from build123d import *

# Parameters (mm, degrees)
SKETCH1_W           = 19.7
SKETCH1_H           = 5.7
SKETCH1_R           = 1.125
BOSS_EXTRUDE1_DEPTH = 0.6
SKETCH2_W           = 10.7
SKETCH2_H           = 5.7
BOSS_EXTRUDE2_DEPTH = 5
SKETCH3_W           = 3.05
SKETCH3_H           = 3.05
BOSS_EXTRUDE3_DEPTH = 7
BOSS_EXTRUDE4_DEPTH = 5


with BuildPart() as part:
    # Sketch1 → Boss-Extrude1 (new body)
    with BuildSketch(Plane.XY):
        with Locations((0, -89.5)):
            Rectangle(SKETCH1_W, SKETCH1_H)
        with Locations((7.5, -89.5)):
            Circle(SKETCH1_R, mode=Mode.SUBTRACT)
        with Locations((-7.5, -89.5)):
            Circle(SKETCH1_R, mode=Mode.SUBTRACT)
    extrude(amount=BOSS_EXTRUDE1_DEPTH)

    # Sketch2 → Boss-Extrude2 (add)
    with BuildSketch(Plane.XY.offset(0.6)):
        with Locations((0, -89.5)):
            Rectangle(SKETCH2_W, SKETCH2_H)
    extrude(amount=BOSS_EXTRUDE2_DEPTH)

    # Sketch3 → Boss-Extrude3 (add)
    with BuildSketch(Plane(origin=(0, 0, 0), x_dir=(-1, 0, 0), z_dir=(0, 0, -1))):
        with Locations((-1.525, -89.5)):
            Rectangle(SKETCH3_W, SKETCH3_H)
    extrude(amount=BOSS_EXTRUDE3_DEPTH)

    # Sketch4 → Boss-Extrude4 (add)
    with BuildSketch(Plane.XY.offset(5.6)):
        with BuildLine():
            Line((-0.5, -89.25), (0.5, -89.25))
            ThreePointArc((0.5, -89.25), (0.75, -89.5), (0.5, -89.75))
            Line((0.5, -89.75), (-0.5, -89.75))
            ThreePointArc((-0.5, -89.75), (-0.75, -89.5), (-0.5, -89.25))
        make_face()
        with BuildLine():
            Line((2, -89.25), (3, -89.25))
            ThreePointArc((3, -89.25), (3.25, -89.5), (3, -89.75))
            Line((3, -89.75), (2, -89.75))
            ThreePointArc((2, -89.75), (1.75, -89.5), (2, -89.25))
        make_face()
        with BuildLine():
            Line((-3, -89.25), (-2, -89.25))
            ThreePointArc((-2, -89.25), (-1.75, -89.5), (-2, -89.75))
            Line((-2, -89.75), (-3, -89.75))
            ThreePointArc((-3, -89.75), (-3.25, -89.5), (-3, -89.25))
        make_face()
    extrude(amount=BOSS_EXTRUDE4_DEPTH)


solid = part.part
Geometry: final body of the model. Coordinates: model frame, mm. A direction names the side the tool comes from. Round coordinates to 2 decimals unless told otherwise and drop trailing zeros. Write each loop counter-clockwise with the first axis right and the second up, starting at its lowest first coordinate (ties: lowest second). Pieces come first, ordered by that corner, then holes. Notation, with made-up numbers: M 33,77 L 87,77 A18 cw 87,108 Z; hole C -14,-39.5 d11. An arc over 180 degrees is marked long. Write item = value, one per line.
Item 1: Section query A-A on x = -7.5. Return loops of the section in (y, z) (3 decimals), then the cut area to 3 significant figures.
Findings:
outline = M -92.35,0 L -90.625,0 L -90.625,0.6 L -92.35,0.6 Z; M -88.375,0 L -86.65,0 L -86.65,0.6 L -88.375,0.6 Z
area = 2.07 mm^2
Item 2: Pin query (flat end, axial travel): P1, Ø4, axis at x = -2.5, z = -4, coming from the +Y side; P2, Ø0.5, axis at x = 2.5, z = 7, coming from the +Y side; P3, Ø2.5, axis at y = -88.5, z = 3.5, coming from the -X side; P4, Ø1.5, axis at x = -7.5, y = -88, coming from the +Z side. Return the tip coordinate at first contact, or that it passes through.
Findings:
P1 = through
P2 = -89.25
P3 = -5.35
P4 = 0.6
Item 3: Access query for faces 1 (the face through (0, -89.25, 8)), 2 (the face through (5.35, -90, 3)), 3 (the face through (-9, -89, 0.6)). Directions: +Z, -Z, +X, -X, +Y, -Y. A direction counts if a zero-diameter tool reaches every point of the face in a straight line with its end or side. Return the directions, or none.
Findings:
face_1 = +Z, +X, -X, +Y
face_2 = +Z, +X, +Y, -Y
face_3 = +Z, -X, +Y, -Y
Item 4: Section query C-C on z = 2.5. Return loops of the section in (x, y), then the cut area to 3 significant figures.
Findings:
outline = M -5.35,-92.35 L 5.35,-92.35 L 5.35,-86.65 L -5.35,-86.65 Z
area = 61.0 mm^2
Item 5: Section query D-D on x = 4. Return loops of the section in (y, z), then the cut area to 3 significant figures.
Findings:
outline = M -92.35,0 L -86.65,0 L -86.65,5.6 L -92.35,5.6 Z
area = 31.9 mm^2
Item 6: Material intervals for line 1 along X through (y, z) = (-89.5, 0.2) (3 decimals); line 2 along Y through (x, z) = (-7.5, 0.4) (3 decimals); line 3 along X through (y, z) = (-89.05, 0.5), sorted ascending. Write a range as [from, to].
Findings:
line_1 = [-9.85, -8.625], [-6.375, 6.375], [8.625, 9.85]
line_2 = [-92.35, -90.625], [-88.375, -86.65]
line_3 = [-9.85, -8.53], [-6.47, 6.47], [8.53, 9.85]
Item 7: Pull-direction query (X, two-part tool) for faces 4 (the face through (0, -90, -3)), 5 (the face through (0, -92.35, 3)), 6 (the face through (-7.74, -90.6, 0.3)); classes: pulls with the +X half, pulls with the -X half, needs draft (parallel to the pull), parting line crosses it, or undercut.
Findings:
face_4 = pulls with the -X half
face_5 = needs draft
face_6 = undercut
Item 8: Section query B-B on y = -87.3. Return loops of the section in (x, z), then the cut area to 3 significant figures.
Findings:
outline = M -9.85,0 L 9.85,0 L 9.85,0.6 L 5.35,0.6 L 5.35,5.6 L -5.35,5.6 L -5.35,0.6 L -9.85,0.6 Z
area = 65.3 mm^2
